from build123d import *

# Parameters (mm, degrees)
EXTRUDE_THIN1_DEPTH = 5


with BuildPart() as part:
    # Sketch1 → Extrude-Thin1 (new, symmetric)
    with BuildSketch(Plane(origin=(0, 0, 0), x_dir=(1, 0, 0), z_dir=(0, 1, 0))):
        with BuildLine():
            Line((-183.400000811, 28), (-183.400000811, 20))
            ThreePointArc((-183.400000811, 20), (-185.161544932, 15.753173798), (-189.411833406, 14))
            Line((-189.411833406, 14), (-696.970447681, 14.999970889))
            ThreePointArc((-696.970447681, 14.999970889), (-711.999422352, -0.131640078), (-696.707182726, -14.997141662))
            Line((-696.707182726, -14.997141662), (-194.526888217, -5.192135604))
            ThreePointArc((-194.526888217, -5.192135604), (-192.341242187, -5.52554921), (-190.393789073, -6.572277241))
            Line((-190.393789073, -6.572277241), (-178.779742807, -15.662291703))
            ThreePointArc((-178.779742807, -15.662291703), (-172, -18.000012126), (-165.220257193, -15.662291703))
            Line((-165.220257193, -15.662291703), (-153.606210927, -6.572277241))
            ThreePointArc((-153.606210927, -6.572277241), (-151.683201757, -5.533765565), (-149.524681207, -5.191333376))
            Line((-149.524681207, -5.191333376), (696.826189088, -14.998992958))
            ThreePointArc((696.826189088, -14.998992958), (711.999796679, -0.078099937), (696.982385781, 14.999989658))
            Line((696.982385781, 14.999989658), (-154.59294936, 14))
            ThreePointArc((-154.59294936, 14), (-158.840146905, 15.75486609), (-160.599999189, 20))
            Line((-160.599999189, 20), (-160.599999189, 28))
            Line((-160.599999189, 28), (-159.099999189, 28))
            Line((-159.099999189, 28), (-159.099999189, 20))
            ThreePointArc((-159.099999189, 20), (-157.780109672, 16.816148836), (-154.594710782, 15.499998966))
            Line((-154.594710782, 15.499998966), (696.980624359, 16.499988624))
            ThreePointArc((696.980624359, 16.499988624), (713.499776346, -0.08590993), (696.808807996, -16.498892254))
            Line((696.808807996, -16.498892254), (-149.542062298, -6.691232672))
            ThreePointArc((-149.542062298, -6.691232672), (-151.202462721, -6.954642048), (-152.681700545, -7.753497183))
            Line((-152.681700545, -7.753497183), (-164.29574681, -16.843511645))
            ThreePointArc((-164.29574681, -16.843511645), (-172, -19.500012126), (-179.70425319, -16.843511645))
            Line((-179.70425319, -16.843511645), (-191.318299455, -7.753497183))
            ThreePointArc((-191.318299455, -7.753497183), (-192.816340312, -6.948321775), (-194.497606489, -6.69184977))
            Line((-194.497606489, -6.69184977), (-696.677900999, -16.496855829))
            ThreePointArc((-696.677900999, -16.496855829), (-713.499364587, -0.144804086), (-696.967492449, 16.499967978))
            Line((-696.967492449, 16.499967978), (-189.408878174, 15.499997089))
            ThreePointArc((-189.408878174, 15.499997089), (-186.221159756, 16.814878288), (-184.900000811, 20))
            Line((-184.900000811, 20), (-184.900000811, 28))
            Line((-184.900000811, 28), (-183.400000811, 28))
        make_face()
    extrude(amount=EXTRUDE_THIN1_DEPTH, both=True)


solid = part.part
Work out the finished part from the listing and answer in its coordinate system (mm). Give positions to 0.01 mm unless a question says otherwise; leave off trailing zeros. Order: outer loops, then holes, each group sorted by start corner. A loop starts at its lowest first (then second) coordinate and runs counter-clockwise, first axis right, second up. Notation, with made-up numbers: M -12,87.25 L 19,87.25 A9 cw 19,91.25 Z; hole C -36.75,-6.5 d3. An arc over 180 degrees is marked long. Return JSON: item names as keys, results as strings.
Q1. Each of these flat-tipped pins is pushed along its axis until it touches: pin 1 (4 mm diameter, centred on y = -0.5, z = -23, fed in from -X); pin 2 (1.5 mm diameter, centred on x = 414, y = -2.5, fed in from +Z); pin 3 (6 mm diameter, centred on y = 1, z = 8.5, fed in from -X). Where does it stop, or does it pass through?
Answer below:
{"pin 1": "stops at x = -184.9", "pin 2": "stops at z = 13.23", "pin 3": "stops at x = -712.56"}
Q2. Find section A-A, the plane x = -592.5. Write down the section's boundary in (y, z).
Answer below:
{"outline": "M -5,-16.29 L 5,-16.29 L 5,-14.79 L -5,-14.79 Z; M -5,12.96 L 5,12.96 L 5,14.46 L -5,14.46 Z"}
Q3. Find section B-B, the plane z = -5.5. Write down the section's boundary in (x, y), and give its area (3 significant figures).
Answer below:
{"outline": "M -712.56,-5 L -710.96,-5 L -710.96,5 L -712.56,5 Z; M 710.96,-5 L 712.56,-5 L 712.56,5 L 710.96,5 Z", "area": "32.0 mm^2"}
Q4. Find the intervals of material crossed by line 1 along X through (y, z) = (-2.5, -19); line 2 along X through (y, z) = (4.75, -0.5); line 3 along Z through (x, y) = (-128, -0.5), in increasing order. Write a range as [from, to].
Answer below:
{"line 1": "x = [-185.01, -183.48], [-160.52, -158.99]", "line 2": "x = [-713.49, -711.99], [711.99, 713.49]", "line 3": "z = [-15.53, -14.03], [5.44, 6.94]"}
